Geometry check sheet. Reference: the model listing, model coordinates, mm. A direction names the side the tool comes from. Coordinates: 2 decimals unless noted, no trailing zeros. Write each loop counter-clockwise with the first axis right and the second up, starting at its lowest first coordinate (ties: lowest second). Pieces come first, ordered by that corner, then holes. Notation, with made-up numbers: M 24,-37 L 80,-37 A23 ccw 80,-23 Z; hole C 19,8.5 d6. An arc over 180 degrees is marked long. Put each result on its own line as item: value. Start each with the question number.
1) Scan lines: line 1 along Z through (x, y) = (-5, -1.75); line 2 along Y through (x, z) = (0.25, -19.5). Record each from-to range of solid material in increasing order.
2) Mould release check, pull along Y, two halves, no side actions. Record for faces 1 (the flat face through (0, 0, -52.5)), 2 (the cylindrical face through (5, 1.6, 3.7)): released by +Y, released by -Y, zero draft, split by the parting line, or undercut.
3) Cross-section at A-A on x = 0. Record the cut outline in (y, z), plus the area to 3 significant figures.
4) Set-up check for faces 3 (the flat face through (-4, -4, 0)), 4 (the cylindrical face through (6, 0, -26)): record each of +Z, -Z, +X, -X, +Y, -Y from which the full face is reachable in a straight line by a thin tool's end or side.
5) Gauge pin test, flat ends, axial feed: pin 1 (6 mm diameter, centred on x = -3.5, z = -44, fed in from +Y); pin 2 (1.5 mm diameter, centred on y = 2.5, z = -2.5, fed in from -X); pin 3 (6 mm diameter, centred on y = 4, z = -4, fed in from -X). Record the tip position at first contact, or that the pin passes through.
6) Cross-section at C-C on z = -48. Record the cut outline in (x, y).
from build123d import *

# Parameters (mm, degrees)
SKETCH_1_R      = 5.25
EXTRUDE_1_DEPTH = 7.5
SKETCH_2_R      = 6
EXTRUDE_2_DEPTH = 42.5
SKETCH_3_R      = 6
EXTRUDE_3_DEPTH = 10


with BuildPart() as part:
    # 草图1 → 凸台-拉伸1 (new body)
    with BuildSketch(Plane.XY):
        Circle(SKETCH_1_R)
    extrude(amount=EXTRUDE_1_DEPTH)

    # 草图2 → 凸台-拉伸2 (add)
    with BuildSketch(Plane(origin=(0, 0, 0), x_dir=(-1, 0, 0), z_dir=(0, 0, -1))):
        Circle(SKETCH_2_R)
    extrude(amount=EXTRUDE_2_DEPTH)

    # 草图3 → 凸台-拉伸3 (add)
    with BuildSketch(Plane(origin=(0, 0, -42.5), x_dir=(-1, 0, 0), z_dir=(0, 0, -1))):
        Circle(SKETCH_3_R)
    extrude(amount=EXTRUDE_3_DEPTH)


solid = part.part
Answer key:
1. line 1: z = -52.5 to 0
1. line 2: y = -5.99 to 5.99
2. face 1: zero draft
2. face 2: split by the parting line
3. outline: M -6,-52.5 L 6,-52.5 L 6,0 L 5.25,0 L 5.25,7.5 L -5.25,7.5 L -5.25,0 L -6,0 Z
3. area: 709 mm²
4. face 3: +Z
4. face 4: +Z, -Z
5. pin 1: stops at y = 5.98
5. pin 2: stops at x = -5.74
5. pin 3: stops at x = -5.92
6. outline: C 0,0 d12
